```python
from build123d import *

# Parameters (mm, degrees)
F0_W     = 279.4
F0_H     = 381
F1_DEPTH = 228.6
F2_T     = -2.54


with BuildPart() as f1:
    # F0 (on Front) → F1 (new body, symmetric)
    with BuildSketch(Plane.XZ):
        Rectangle(F0_W, F0_H)
    extrude(amount=F1_DEPTH, both=True)

    # F2
    f2_openings = [f1.faces().sort_by_distance(p)[0] for p in [
        (-139.7, 0, 0),
    ]]
    offset(amount=F2_T, openings=f2_openings)


solid = f1.part
```
Verification items for the finished model (mm, model axes). A direction names the side the tool comes from. Coordinates: 2 decimals unless noted, no trailing zeros. Write each loop counter-clockwise with the first axis right and the second up, starting at its lowest first coordinate (ties: lowest second). Pieces come first, ordered by that corner, then holes. Notation, with made-up numbers: M 83.5,11.25 L 87.5,11.25 A17 ccw 87.5,29.25 Z; hole C -5.5,-13 d8. An arc over 180 degrees is marked long. One line per item, written item: value.
Item 1: Gauge pin test, flat end, axial feed: pin 1 Ø10 at (y, z) = (39.5, 109) entering from -X. Record the tip position at first contact, or that the pin passes through.
Check sheet entries:
pin 1: stops at x = 137.16
Item 2: Scan lines: line 1 along Z through (x, y) = (-21, -100); line 2 along Y through (x, z) = (15, -136.5); line 3 along X through (y, z) = (9, 91.5). Record each from-to range of solid material in increasing order.
Check sheet entries:
line 1: z = -190.5 to -187.96, 187.96 to 190.5
line 2: y = -228.6 to -226.06, 226.06 to 228.6
line 3: x = 137.16 to 139.7
Item 3: Section check B-B, the plane z = 117. Record the boundary of the cut face in (x, y), plus the area to 3 significant figures.
Check sheet entries:
outline: M -139.7,-228.6 L 139.7,-228.6 L 139.7,228.6 L -139.7,228.6 L -139.7,226.06 L 137.16,226.06 L 137.16,-226.06 L -139.7,-226.06 Z
area: 2,570 mm^2
Item 4: Section check C-C, the plane y = 180.5. Record the boundary of the cut face in (x, z).
Check sheet entries:
outline: M -139.7,-190.5 L 139.7,-190.5 L 139.7,190.5 L -139.7,190.5 L -139.7,187.96 L 137.16,187.96 L 137.16,-187.96 L -139.7,-187.96 Z
Item 5: Access from +Z, -Z, +X, -X, +Y, -Y to the whole of each face (thin tool, end or side, straight path). Record for faces 1 (the flat face through (-3, 226.06, 3)), 2 (the flat face through (-2, -3, 190.5)).
Check sheet entries:
face 1: -X
face 2: +Z, +X, -X, +Y, -Y
Item 6: Mould release check, pull along Y, two halves, no side actions. Record for faces 3 (the flat face through (-2, 228.6, 3)), 4 (the flat face through (-3, -3, -187.96)), 5 (the flat face through (-2, -3, -190.5)): pulls with the +Y half, pulls with the -Y half, needs draft (parallel to the pull), parting line crosses it, or undercut.
Check sheet entries:
face 3: pulls with the +Y half
face 4: undercut
face 5: needs draft
Item 7: Section check A-A, the plane x = 82. Record the boundary of the cut face in (y, z).
Check sheet entries:
outline: M -228.6,-190.5 L 228.6,-190.5 L 228.6,190.5 L -228.6,190.5 Z; hole M -226.06,-187.96 L 226.06,-187.96 L 226.06,187.96 L -226.06,187.96 Z
